```python
from build123d import *

# Parameters (mm, degrees)
SKETCH1_W           = 300
SKETCH1_H           = 200
BOSS_EXTRUDE1_DEPTH = 20
SKETCH2_W           = 12.2
SKETCH2_H           = 4
CUT_EXTRUDE1_DEPTH  = 317.859590355
LPATTERN1_COUNT     = 9
LPATTERN1_PITCH     = 15.300152


with BuildPart() as part:
    # Sketch1 → Boss-Extrude1 (new body)
    with BuildSketch(Plane(origin=(0, 0, 0), x_dir=(1, 0, 0), z_dir=(0, 1, 0))):
        Rectangle(SKETCH1_W, SKETCH1_H)
    extrude(amount=-BOSS_EXTRUDE1_DEPTH)

    # Sketch2 → Cut-Extrude1 (cut, through all)
    with BuildSketch(Plane(origin=(150, 0, 0), x_dir=(0, 0, -1), z_dir=(1, 0, 0))):
        with Locations((-61.200608, -2)):
            Rectangle(SKETCH2_W, SKETCH2_H)
    cut_extrude1 = extrude(amount=-CUT_EXTRUDE1_DEPTH, mode=Mode.SUBTRACT)

    # LPattern1: Cut-Extrude1 ×9
    with Locations(*[(0, 0, -i * LPATTERN1_PITCH) for i in range(1, LPATTERN1_COUNT)]):
        add(cut_extrude1, mode=Mode.SUBTRACT)


solid = part.part
```
For this review, take the finished solid that the model builds, in its own axes (mm). A direction names the side the tool comes from. Round coordinates to 2 decimals unless told otherwise and drop trailing zeros. Write each loop counter-clockwise with the first axis right and the second up, starting at its lowest first coordinate (ties: lowest second). Pieces come first, ordered by that corner, then holes. Notation, with made-up numbers: (26, -17) - (52, -17) arc R14 cw to (52, -4) - close; hole circle Ø10 at (55.5, 65.5). An arc over 180 degrees is marked (long way). Put each result on its own line as item: value.
Q1. We need section A-A (z = -31). Give the boundary of the cut face in (x, y), and give its area (3 significant figures).
Solved:
outline: (-150, -20) - (150, -20) - (150, -4) - (-150, -4) - close
area: 4,800 mm2
Q2. Mouldability with a two-part tool opening along Z and no side actions: class faces 1 (the face through (-2, 0, -84)), 2 (the face through (-2, -10, -100)), 3 (the face through (-2, -10, 100)), 4 (the face through (2, -4, 46)) as released by +Z, released by -Z, zero draft, split by the parting line, or undercut.
Solved:
face 1: zero draft
face 2: released by -Z
face 3: released by +Z
face 4: undercut
Q3. Insertion check: pin 1 Ø8 at (x, z) = (-77, 47) entering from +Y. The pin has a flat end and moves straight along its axis. Give the tip position at first contact, or say it passes through.
Solved:
pin 1: stops at y = -4
Q4. Wall thickness on probe 1 along Y at (x, z) = (-57, -15): over which ranges is the line inside the solid? List them lowest first.
Solved:
probe 1: y = -20 to -4
Q5. Machinability: for faces 5 (the face through (2, -4, 31)), 6 (the face through (-2, -20, -1)), which of the approach directions +Z, -Z, +X, -X, +Y, -Y give a long, thin tool a straight path to every point of the face, cutting with its end or side? Answer none if there is none.
Solved:
face 5: +X, -X, +Y
face 6: +Z, -Z, +X, -X, -Y
